from build123d import *
from build123d.topology import SkipClean

# Parameters (mm, degrees)
BOSS_EXTRUDE1_DEPTH = 3.175
BOSS_EXTRUDE2_START = 3.175
SKETCH2_R           = 3.175
BOSS_EXTRUDE2_DEPTH = 3.175
SKETCH3_R           = 4.7625
BOSS_EXTRUDE3_DEPTH = 6.35
BOSS_EXTRUDE4_START = 3.175
SKETCH4_R           = 4.7625
BOSS_EXTRUDE4_DEPTH = 3.175
CUT_EXTRUDE1_START  = -4.0894
CUT_EXTRUDE1_DEPTH  = 4.0894
SKETCH6_W           = 0.762
SKETCH6_H           = 1.27
CUT_EXTRUDE2_DEPTH  = 9.525


with BuildPart() as part:
    # Sketch1 → Boss-Extrude1 (new body)
    with BuildSketch(Plane.XY):
        with BuildLine():
            Line((11.017558073, 1.449506939), (7.869684338, 25.3761821))
            ThreePointArc((7.869684338, 25.3761821), (7.920527939, 24.859610334), (7.9375, 24.34082))
            ThreePointArc((7.9375, 24.34082), (5.612660076, 18.728159924), (0, 16.40332))
            Line((0, 16.40332), (0, 11.1125))
            ThreePointArc((0, 11.1125), (7.327346395, 8.354498851), (11.017558073, 1.449506939))
        make_face()
        with BuildLine():
            ThreePointArc((7.9375, 24.34082), (7.920527939, 24.859610334), (7.869684338, 25.3761821))
            ThreePointArc((7.869684338, 25.3761821), (5.233818854, 30.30831918), (0, 32.27832))
            Line((0, 32.27832), (0, 29.10332))
            ThreePointArc((0, 29.10332), (3.367596045, 27.708416045), (4.7625, 24.34082))
            ThreePointArc((4.7625, 24.34082), (3.367596045, 20.973223955), (0, 19.57832))
            Line((0, 19.57832), (0, 16.40332))
            ThreePointArc((0, 16.40332), (5.612660076, 18.728159924), (7.9375, 24.34082))
        make_face()
        with BuildLine():
            Line((0, 29.10332), (0, 32.27832))
            ThreePointArc((0, 32.27832), (-5.233818854, 30.30831918), (-7.869684338, 25.3761821))
            ThreePointArc((-7.869684338, 25.3761821), (-5.96749918, 19.107001146), (0, 16.40332))
            Line((0, 16.40332), (0, 19.57832))
            ThreePointArc((0, 19.57832), (-4.7625, 24.34082), (0, 29.10332))
        make_face()
        with BuildLine():
            ThreePointArc((-11.017558073, 1.449506939), (-7.327346395, 8.354498851), (0, 11.1125))
            Line((0, 11.1125), (0, 16.40332))
            ThreePointArc((0, 16.40332), (-5.96749918, 19.107001146), (-7.869684338, 25.3761821))
            Line((-7.869684338, 25.3761821), (-11.017558073, 1.449506939))
        make_face()
        with BuildLine():
            ThreePointArc((11.1125, 0), (11.088739115, 0.726306467), (11.017558073, 1.449506939))
            ThreePointArc((11.017558073, 1.449506939), (7.327346395, 8.354498851), (0, 11.1125))
            Line((0, 11.1125), (0, 4.7625))
            ThreePointArc((0, 4.7625), (3.367596045, 3.367596045), (4.7625, 0))
            ThreePointArc((4.7625, 0), (3.367596045, -3.367596045), (0, -4.7625))
            Line((0, -4.7625), (0, -11.1125))
            ThreePointArc((0, -11.1125), (7.327346395, -8.354498851), (11.017558073, -1.449506939))
            ThreePointArc((11.017558073, -1.449506939), (11.088739115, -0.726306467), (11.1125, 0))
        make_face()
        with BuildLine():
            Line((0, 4.7625), (0, 11.1125))
            ThreePointArc((0, 11.1125), (-7.327346395, 8.354498851), (-11.017558073, 1.449506939))
            ThreePointArc((-11.017558073, 1.449506939), (-11.1125, 0), (-11.017558073, -1.449506939))
            ThreePointArc((-11.017558073, -1.449506939), (-7.327346395, -8.354498851), (0, -11.1125))
            Line((0, -11.1125), (0, -4.7625))
            ThreePointArc((0, -4.7625), (-4.7625, 0), (0, 4.7625))
        make_face()
        with BuildLine():
            Line((7.869684338, -25.3761821), (11.017558073, -1.449506939))
            ThreePointArc((11.017558073, -1.449506939), (7.327346395, -8.354498851), (0, -11.1125))
            Line((0, -11.1125), (0, -16.40332))
            ThreePointArc((0, -16.40332), (5.612660076, -18.728159924), (7.9375, -24.34082))
            ThreePointArc((7.9375, -24.34082), (7.920527939, -24.859610334), (7.869684338, -25.3761821))
        make_face()
        with BuildLine():
            Line((0, -16.40332), (0, -11.1125))
            ThreePointArc((0, -11.1125), (-7.327346395, -8.354498851), (-11.017558073, -1.449506939))
            Line((-11.017558073, -1.449506939), (-7.869684338, -25.3761821))
            ThreePointArc((-7.869684338, -25.3761821), (-5.96749918, -19.107001146), (0, -16.40332))
        make_face()
        with BuildLine():
            ThreePointArc((0, -32.27832), (5.233818854, -30.30831918), (7.869684338, -25.3761821))
            ThreePointArc((7.869684338, -25.3761821), (7.920527939, -24.859610334), (7.9375, -24.34082))
            ThreePointArc((7.9375, -24.34082), (5.612660076, -18.728159924), (0, -16.40332))
            Line((0, -16.40332), (0, -19.57832))
            ThreePointArc((0, -19.57832), (3.367596045, -20.973223955), (4.7625, -24.34082))
            ThreePointArc((4.7625, -24.34082), (3.367596045, -27.708416045), (0, -29.10332))
            Line((0, -29.10332), (0, -32.27832))
        make_face()
        with BuildLine():
            ThreePointArc((-7.869684338, -25.3761821), (-5.233818854, -30.30831918), (0, -32.27832))
            Line((0, -32.27832), (0, -29.10332))
            ThreePointArc((0, -29.10332), (-4.7625, -24.34082), (0, -19.57832))
            Line((0, -19.57832), (0, -16.40332))
            ThreePointArc((0, -16.40332), (-5.96749918, -19.107001146), (-7.869684338, -25.3761821))
        make_face()
    extrude(amount=BOSS_EXTRUDE1_DEPTH)

    # Sketch2 → Boss-Extrude2 (add)
    with BuildSketch(Plane(origin=(0, 0, 0), x_dir=(-1, 0, 0), z_dir=(0, 0, -1)).offset(BOSS_EXTRUDE2_START)):
        with BuildLine():
            Line((-9.955119086, 9.525), (9.955119086, 9.525))
            Line((9.955119086, 9.525), (11.017558073, 1.449506939))
            ThreePointArc((11.017558073, 1.449506939), (11.1125, 0), (11.017558073, -1.449506939))
            Line((11.017558073, -1.449506939), (9.955119086, -9.525))
            Line((9.955119086, -9.525), (-9.955119086, -9.525))
            Line((-9.955119086, -9.525), (-11.017558073, -1.449506939))
            ThreePointArc((-11.017558073, -1.449506939), (-11.1125, 0), (-11.017558073, 1.449506939))
            Line((-11.017558073, 1.449506939), (-9.955119086, 9.525))
        make_face()
        Circle(SKETCH2_R, mode=Mode.SUBTRACT)
    extrude(amount=-BOSS_EXTRUDE2_DEPTH)

    # Sketch3 → Boss-Extrude3 (add)
    with SkipClean():  # the faces are left unmerged after this step: merging them gives an invalid solid
        with BuildSketch(Plane.XY.offset(3.175)):
            with BuildLine():
                Line((-9.955119086, 9.525), (9.955119086, 9.525))
                Line((9.955119086, 9.525), (11.017558073, 1.449506939))
                ThreePointArc((11.017558073, 1.449506939), (11.1125, 0), (11.017558073, -1.449506939))
                Line((11.017558073, -1.449506939), (9.955119086, -9.525))
                Line((9.955119086, -9.525), (-9.955119086, -9.525))
                Line((-9.955119086, -9.525), (-11.017558073, -1.449506939))
                ThreePointArc((-11.017558073, -1.449506939), (-11.1125, 0), (-11.017558073, 1.449506939))
                Line((-11.017558073, 1.449506939), (-9.955119086, 9.525))
            make_face()
            Circle(SKETCH3_R, mode=Mode.SUBTRACT)
        extrude(amount=BOSS_EXTRUDE3_DEPTH)

    # Sketch4 → Boss-Extrude4 (add)
    # profile 1 of 2: a face of its own
    with SkipClean():  # the faces are left unmerged after this step: merging them gives an invalid solid
        with BuildSketch(Plane(origin=(0, 0, 0), x_dir=(-1, 0, 0), z_dir=(0, 0, -1)).offset(BOSS_EXTRUDE4_START)):
            with BuildLine():
                Line((9.955119086, 9.525), (-9.955119086, 9.525))
                Line((-9.955119086, 9.525), (-7.869684338, 25.3761821))
                ThreePointArc((-7.869684338, 25.3761821), (0, 32.27832), (7.869684338, 25.3761821))
                Line((7.869684338, 25.3761821), (9.955119086, 9.525))
            make_face()
            with Locations(Location((0, 24.34082, 0), (0, 0, 180))):
                Circle(SKETCH4_R, mode=Mode.SUBTRACT)
        # profile 2 of 2: a face of its own
        with BuildSketch(Plane(origin=(0, 0, 0), x_dir=(-1, 0, 0), z_dir=(0, 0, -1)).offset(BOSS_EXTRUDE4_START)):
            with BuildLine():
                Line((-9.955119086, -9.525), (-7.869684338, -25.3761821))
                ThreePointArc((-7.869684338, -25.3761821), (0, -32.27832), (7.869684338, -25.3761821))
                Line((7.869684338, -25.3761821), (9.955119086, -9.525))
                Line((9.955119086, -9.525), (-9.955119086, -9.525))
            make_face()
            with Locations(Location((0, -24.34082, 0), (0, 0, 180))):
                Circle(SKETCH4_R, mode=Mode.SUBTRACT)
        extrude(amount=-BOSS_EXTRUDE4_DEPTH)

    # Sketch5 → Cut-Extrude1 (cut)
    with SkipClean():  # the faces are left unmerged after this step: merging them gives an invalid solid
        with BuildSketch(Plane.XY.offset(3.175).offset(CUT_EXTRUDE1_START)):
            with BuildLine():
                Line((-7.869684338, -25.3761821), (-9.955119086, -9.525))
                Line((-9.955119086, -9.525), (9.955119086, -9.525))
                Line((9.955119086, -9.525), (7.869684338, -25.3761821))
                ThreePointArc((7.869684338, -25.3761821), (0, -32.27832), (-7.869684338, -25.3761821))
            make_face()
            with BuildLine():
                Line((-7.869684338, 25.3761821), (-9.955119086, 9.525))
                Line((-9.955119086, 9.525), (9.955119086, 9.525))
                Line((9.955119086, 9.525), (7.869684338, 25.3761821))
                ThreePointArc((7.869684338, 25.3761821), (0, 32.27832), (-7.869684338, 25.3761821))
            make_face()
        extrude(amount=CUT_EXTRUDE1_DEPTH, mode=Mode.SUBTRACT)

    # Sketch6 → Cut-Extrude2 (cut)
    with SkipClean():  # the faces are left unmerged after this step: merging them gives an invalid solid
        with BuildSketch(Plane.XY.offset(9.525)):
            with Locations((-4.7625, 0)):
                Rectangle(SKETCH6_W, SKETCH6_H)
        extrude(amount=-CUT_EXTRUDE2_DEPTH, mode=Mode.SUBTRACT)


solid = part.part
Build history of the part. All positions in model axes, mm. A direction names the side the tool comes from. Round coordinates to 2 decimals unless told otherwise and drop trailing zeros. Write each loop counter-clockwise with the first axis right and the second up, starting at its lowest first coordinate (ties: lowest second). Pieces come first, ordered by that corner, then holes. Notation, with made-up numbers: (-40, 39.25) -> (-18, 39.25) arc R10 cw to (-18, 48.25) -> close; hole circle Ø7 at (29.25, 37.5). An arc over 180 degrees is marked (long way). Write item = value, one per line.
(1) Probe L1, parallel to Y at x = 0, z = -0.65 (3 decimals); L2, parallel to Y at x = 0.25, z = 6.75 (3 decimals); L3, parallel to Z at x = 8, y = -12 (3 decimals). List the from-to ranges inside material, lowest first.
Answer:
L1 = -9.525 to -3.175, 3.175 to 9.525
L2 = -9.525 to -4.756, 4.756 to 9.525
L3 = -3.175 to -0.914
(2) Band-saw the part on B-B (z = 7). Give the cut face in (x, y) (1 decimal), then the cut area to 3 significant figures.
Answer:
outline = (-11, -1.4) -> (-10, -9.5) -> (10, -9.5) -> (11, -1.4) arc R11.1 ccw to (11, 1.4) -> (10, 9.5) -> (-10, 9.5) -> (-11, 1.4) arc R11.1 ccw to start; hole (-5.1, -0.6) -> (-4.7, -0.6) arc R4.8 ccw (long way) to (-4.7, 0.6) -> (-5.1, 0.6) -> close
area = 331 mm2
(3) Band-saw the part on C-C (y = -22). Give the cut face in (x, z) (3 decimals), then the cut area to 3 significant figures.
Answer:
outline = (-8.314, -3.175) -> (-4.148, -3.175) -> (-4.148, -0.914) -> (-8.314, -0.914) -> close; (4.148, -3.175) -> (8.314, -3.175) -> (8.314, -0.914) -> (4.148, -0.914) -> close
area = 18.8 mm2
(4) Band-saw the part on A-A (x = 1.75). Give the cut face in (y, z) (1 decimal).
Answer:
outline = (-32.1, -3.2) -> (-28.8, -3.2) -> (-28.8, -0.9) -> (-32.1, -0.9) -> close; (-19.9, -3.2) -> (-2.6, -3.2) -> (-2.6, 0) -> (-4.4, 0) -> (-4.4, 9.5) -> (-9.5, 9.5) -> (-9.5, -0.9) -> (-19.9, -0.9) -> close; (2.6, -3.2) -> (19.9, -3.2) -> (19.9, -0.9) -> (9.5, -0.9) -> (9.5, 9.5) -> (4.4, 9.5) -> (4.4, 0) -> (2.6, 0) -> close; (28.8, -3.2) -> (32.1, -3.2) -> (32.1, -0.9) -> (28.8, -0.9) -> close
(5) Tool access for faces 4 (the face through (0.84, 3.24, 0)), 5 (the face through (0, 9.525, 4)), 6 (the face through (0, -18, -0.914)): list every direction of +Z, -Z, +X, -X, +Y, -Y with a clear straight run to the whole face (end or side of a thin tool).
Answer:
face_4 = +Z
face_5 = +Z, +X, -X, +Y
face_6 = +Z, +X, -X, -Y
(6) Band-saw the part on D-D (z = -2.5). State how many separate pieces and enclosed holes the cut face has, then the cut area to 3 significant figures.
Answer:
separate_pieces = 1
enclosed_holes = 3
area = 959 mm2
(7) Two-plate mould, pull along X, no slides. Class faces 1 (the face through (3, 4, 9.525)), 2 (the face through (-5.144, 0, 5)), 3 (the face through (0.16, 32.277, -2.061)): pulls with the +X half, pulls with the -X half, needs draft (parallel to the pull), parting line crosses it, or undercut.
Answer:
face_1 = needs draft
face_2 = undercut
face_3 = parting line crosses it
(8) Flat gauge pins, fed straight in: pin 1 (7.5 mm diameter, centred on x = -2, y = -1, fed in from +Z) (3 decimals); pin 2 (2 mm diameter, centred on x = 0, y = 17.5, fed in from +Z); pin 3 (0.5 mm diameter, centred on x = -5, z = 6.5, fed in from +Y) (3 decimals); pin 4 (1.5 mm diameter, centred on x = 5, z = 4.5, fed in from -Y) (3 decimals). Where does each tip first touch, or does it go through?
Answer:
pin_1 = 9.525
pin_2 = -0.91
pin_3 = 9.525
pin_4 = -9.525
